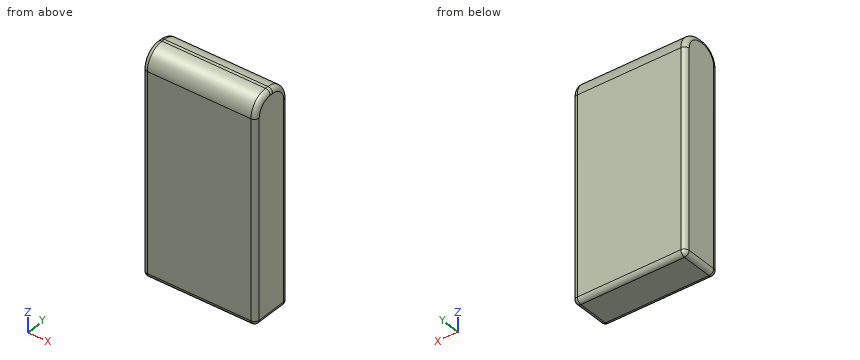
Autodesk Inventor part; units mm, degrees
ref_plane "YZ Plane" through (0, 0, 0) normal (1, 0, 0) x (0, 1, 0)
ref_plane "XZ Plane" through (0, 0, 0) normal (0, 1, 0) x (-1, 0, 0)
ref_plane "XY Plane" through (0, 0, 0) normal (0, 0, 1) x (1, 0, 0)
sketch "Sketch1" plane through (0, 0, 0) normal (0, 1, 0) x (-1, 0, 0)
  line L0 (0, 0) -> (36, 0)
  line L1 (36, 0) -> (36, -70)
  line L2 (36, -70) -> (0, -70)
  line L3 (0, -70) -> (0, 0)
  dimension "d0" = 36
  dimension "d1" = 70
extrude "Extrusion1" add sketch "Sketch1" along normal blind 13
fillet "Fillet1" radius 6 2 edges at (-18, 13, 0) (-18, 0, 0)
fillet "Fillet2" radius 1.5 14 edges at (0, 11.2426, -1.7574) (0, 6.5, 0) (0, 1.7574, -1.7574) (0, 0, -38) (0, 13, -38) (-36, 11.2426, -1.7574) (-36, 6.5, 0) (-36, 1.7574, -1.7574) (-36, 0, -38) (-36, 13, -38) (0, 6.5, -70) (-18, 13, -70) (-36, 6.5, -70) (-18, 0, -70)
properties part number "LIPO 1050"
Here's how the part is built. I have some questions about the finished solid (model axes, mm). Coordinates: 2 decimals unless noted, no trailing zeros. Order: outer loops, then holes, each group sorted by start corner. A loop starts at its lowest first (then second) coordinate and runs counter-clockwise, first axis right, second up.
Item 1: I'm going to push a flat-ended pin straight in: pin 1 Ø2 at (x, z) = (-22, -36.5) entering from -Y. Where does the tip first touch, or does it pass through?
Response values:
pin 1: stops at y = 0
Item 2: I need wall thicknesses on probe 1 along Z at (x, y) = (-25.5, 7.25); probe 2 along Z at (x, y) = (-1.5, 4); probe 3 along X at (y, z) = (12.25, -49.5). Which ranges of each line are inside material? Lowest first, please.
Response values:
probe 1: z = -70 to -0.01
probe 2: z = -70 to -0.34
probe 3: x = -35.8 to -0.2
Item 3: If we section it at A-A, the plane x = -12: List the corners of the cut face in (y, z) for me.
Response values:
outline: (0, -68.5) arc R1.5 ccw to (1.5, -70) - (11.5, -70) arc R1.5 ccw to (13, -68.5) - (13, -6) arc R6 ccw to (7, 0) - (6, 0) arc R6 ccw to (0, -6) - close
